from build123d import *

# Parameters (mm, degrees)
F0_R     = 3
F1_DEPTH = 5


with BuildPart() as f1:
    # F0 (on Top) → F1 (new body)
    with BuildSketch(Plane.XY):
        with BuildLine():
            ThreePointArc((42.182817, -18.346934), (-45.745768, -4.82957), (37.42163, 26.751105))
            ThreePointArc((37.42163, 26.751105), (39.20213, 25.212564), (41.489198, 24.658834))
            Line((41.489198, 24.658834), (48.676006, 24.658834))
            ThreePointArc((48.676006, 24.658834), (53.035379, 27.210188), (52.945831, 32.260486))
            ThreePointArc((52.945831, 32.260486), (30.363217, 54.056221), (0, 62))
            Line((0, 62), (-58.927971, 62))
            ThreePointArc((-58.927971, 62), (-62.463505, 60.535534), (-63.927971, 57))
            Line((-63.927971, 57), (-63.927971, -48))
            ThreePointArc((-63.927971, -48), (-62.463505, -51.535534), (-58.927971, -53))
            Line((-58.927971, -53), (-33.54102, -53))
            ThreePointArc((-33.54102, -53), (-32.245217, -53.170829), (-31.037958, -53.671642))
            ThreePointArc((-31.037958, -53.671642), (20.722466, -58.434402), (57.917728, -22.125478))
            ThreePointArc((57.917728, -22.125478), (57.36529, -17.505814), (53.246943, -15.341166))
            Line((53.246943, -15.341166), (46.767905, -15.341166))
            ThreePointArc((46.767905, -15.341166), (44.026661, -16.159589), (42.182817, -18.346934))
        make_face()
        with Locations((-51.826652, -39.644886)):
            Circle(F0_R, mode=Mode.SUBTRACT)
        with Locations((48.010073, -26.615358)):
            Circle(F0_R, mode=Mode.SUBTRACT)
        with Locations((-52.489314, 50.138593)):
            Circle(F0_R, mode=Mode.SUBTRACT)
        with Locations((42.842665, 34.981498)):
            Circle(F0_R, mode=Mode.SUBTRACT)
    extrude(amount=F1_DEPTH)


solid = f1.part
CAD build for the part. Positions are in the model's coordinates, mm. A direction names the side the tool comes from. Round coordinates to 2 decimals unless told otherwise and drop trailing zeros. Write each loop counter-clockwise with the first axis right and the second up, starting at its lowest first coordinate (ties: lowest second). Pieces come first, ordered by that corner, then holes. Notation, with made-up numbers: M -15,-16.5 L 26,-16.5 A22 cw 26,14.5 Z; hole C -18.5,75 d11. An arc over 180 degrees is marked long. Use a Markdown table: item, result. Add a question column.
1. Drill centre lines: probe 1 along Y at (x, z) = (0.5, 2.55); probe 2 along X at (y, z) = (-40, 0.6); probe 3 along Y at (x, z) = (47, 4.8). Where is each one in solid material? Low to high.
2. Slice it at B-B on z = 1.4. Give the cut face in (x, y).
3. Slice it at C-C on y = 0. Give the cut face in (x, z), then the cut area to 3 significant figures.
4. Pull direction X, two halves, no side cores. Call faces 4 (the face through (-49.055, -40.794, 2.465)), 5 (the face through (-46, -53, 2)), 6 (the face through (20.013, -58.681, 2.465)): released by +X, released by -X, zero draft, split by the parting line, or undercut.
5. Slice it at A-A on x = 5. Give the cut face in (y, z).
6. Flat gauge pins, fed straight in: P1, Ø1.5, axis at x = -52, z = 2.5, coming from the -Y side; P2, Ø2, axis at x = 7, z = 1.5, coming from the +Y side; P3, Ø1.5, axis at x = 44, z = 2.5, coming from the -Y side; P4, Ø8, axis at x = -51.83, y = -39.64, coming from the +Z side. Where does each tip first touch, or does it go through?
7. 3-axis set-ups, long thin cutter, end or side, ignore diameter. For faces 1 (the face through (44.06, -16.14, 2.46)), 2 (the face through (45, 24.659, 2)), 3 (the face through (-62.4, 60.6, 2.5)): which of +Z, -Z, +X, -X, +Y, -Y reach the whole face in a straight line?
Reply:
| question | item | result |
|---|---|---|
| 1 | probe 1 | y = -62 to -46, 46 to 62 |
| 1 | probe 2 | x = -63.93 to -54.81, -48.85 to -22.72, 22.72 to 47.37 |
| 1 | probe 3 | y = -40.44 to -29.44, -23.79 to -15.34, 24.66 to 40.44 |
| 2 | outline | M -63.93,-48 A5 ccw -58.93,-53 L -33.54,-53 A5 cw -31.04,-53.67 A62 ccw 57.92,-22.13 A5 ccw 53.25,-15.34 L 46.77,-15.34 A5 ccw 42.18,-18.35 A46 cw long 37.42,26.75 A5 ccw 41.49,24.66 L 48.68,24.66 A5 ccw 52.95,32.26 A62 ccw 0,62 L -58.93,62 A5 ccw -63.93,57 Z; hole C -52.49,50.14 d6; hole C -51.83,-39.64 d6; hole C 42.84,34.98 d6; hole C 48.01,-26.62 d6 |
| 3 | outline | M -63.93,0 L -46,0 L -46,5 L -63.93,5 Z |
| 3 | area | 89.6 mm^2 |
| 4 | face 4 | undercut |
| 4 | face 5 | zero draft |
| 4 | face 6 | split by the parting line |
| 5 | outline | M -61.8,0 L -45.73,0 L -45.73,5 L -61.8,5 Z; M 45.73,0 L 61.8,0 L 61.8,5 L 45.73,5 Z |
| 6 | P1 | stops at y = -53 |
| 6 | P2 | stops at y = 61.71 |
| 6 | P3 | stops at y = -44.42 |
| 6 | P4 | stops at z = 5 |
| 7 | face 1 | +Z, -Z |
| 7 | face 2 | +Z, -Z, +X |
| 7 | face 3 | +Z, -Z, -X, +Y |
